Design review of the part built by this model. Coordinates are the model's own, in mm. Face numbers are marked on the shaded views. Coordinates: 2 decimals unless noted, no trailing zeros. Loops run counter-clockwise (first coordinate to the right, second up) from the corner with the lowest first, then second, coordinate; pieces in that order, holes last.
Q1. Wall thickness on probe 1 along X at (y, z) = (14.2, 0); probe 2 along Y at (x, z) = (13, 10.5); probe 3 along X at (y, z) = (11.05, -27.5): over which ranges is each line inside the solid? List them lowest first.
Q2. Add section D-D on x = -27.5. Give the boundary of the cut face in (y, z), and give its area (3 significant figures).
Q3. Add section B-B on x = 0. Give the boundary of the cut face in (y, z), and give its area (4 significant figures).
Q4. Add section A-A on z = -27.5. Give the boundary of the cut face in (x, y), and give its area (3 significant figures).
Q5. For P1, Ø4, axis at x = 0, z = 27.5, coming from the -Y side; P2, Ø1.5, axis at y = 2.5, z = -17.5, coming from the +X side; P3, Ø12, axis at x = 8, z = -24.5, coming from the +Y side, all flat-tipped, find the tip position at first contact; note any pin that passes through.
Q6. Draft analysis for pull direction Z (two halves, no side actions). For the marked faces 1 and 2, state which applies: released by +Z, released by -Z, zero draft, split by the parting line, or undercut.
Q7. Add section C-C on z = 0. Give the boundary of the cut face in (x, y), and give its area (4 significant figures).
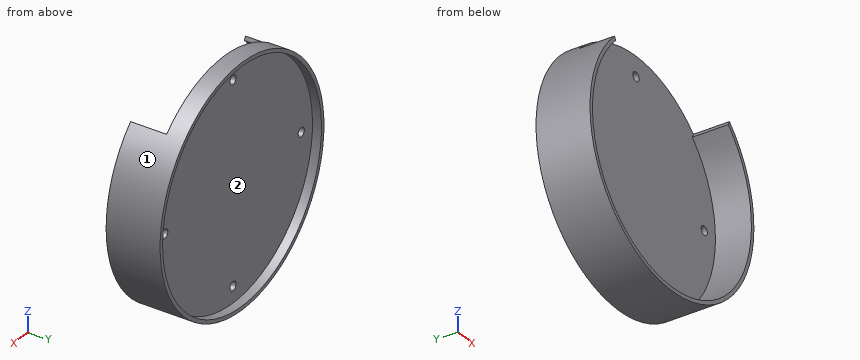
```python
from build123d import *

# Parameters (mm, degrees)
SKETCH1_R               = 33
SKETCH1_R_2             = 1.25
BOSS_EXTRUDE1_DEPTH     = 12.5
SKETCH2_R               = 32
CUT_EXTRUDE2_DEPTH      = 10
SKETCH8_R               = 33
SKETCH8_R_2             = 32
BOSS_EXTRUDE2_DEPTH     = 15
CUT_REVOLVE_THIN2_DEPTH = 10


# Read off the part's stored shape, not the designer's step: Cut-Revolve-Thin2
with BuildPart() as part:
    # Sketch1 → Boss-Extrude1 (new body)
    with BuildSketch(Plane(origin=(0, 0, 0), x_dir=(1, 0, 0), z_dir=(0, 1, 0))):
        with Locations(Location((0, 0, 0), (0, 0, 270))):
            Circle(SKETCH1_R)
        with Locations(Location((0, 27.5, 0), (0, 0, 270))):
            Circle(SKETCH1_R_2, mode=Mode.SUBTRACT)
        with Locations(Location((27.5, 0, 0), (0, 0, 270))):
            Circle(SKETCH1_R_2, mode=Mode.SUBTRACT)
        with Locations(Location((0, -27.5, 0), (0, 0, 270))):
            Circle(SKETCH1_R_2, mode=Mode.SUBTRACT)
        with Locations(Location((-27.5, 0, 0), (0, 0, 270))):
            Circle(SKETCH1_R_2, mode=Mode.SUBTRACT)
    extrude(amount=BOSS_EXTRUDE1_DEPTH)

    # Sketch2 → Cut-Extrude2 (cut)
    with BuildSketch(Plane(origin=(0, 0, 0), x_dir=(1, 0, 0), z_dir=(0, 1, 0))):
        with Locations(Location((0, 0, 0), (0, 0, 270))):
            Circle(SKETCH2_R)
    extrude(amount=CUT_EXTRUDE2_DEPTH, mode=Mode.SUBTRACT)

    # Sketch8 → Boss-Extrude2 (add)
    with BuildSketch(Plane(origin=(0, 0, 0), x_dir=(1, 0, 0), z_dir=(0, 1, 0))):
        with Locations(Location((0, 0, 0), (0, 0, 270))):
            Circle(SKETCH8_R)
        with Locations(Location((0, 0, 0), (0, 0, 270))):
            Circle(SKETCH8_R_2, mode=Mode.SUBTRACT)
    extrude(amount=BOSS_EXTRUDE2_DEPTH)

    # Cut-Revolve-Thin2 outline → Cut-Revolve-Thin2 (cut)
    with BuildSketch(Plane(origin=(0, 0, 0), x_dir=(1, 0, 0), z_dir=(0, 1, 0))):
        with BuildLine():
            ThreePointArc((-22.709083631, -22.545454545), (-22.928374212, -23.0355805), (-23.137087961, -23.53030303))
            ThreePointArc((-23.137087961, -23.53030303), (0, -33), (23.137087961, -23.53030303))
            ThreePointArc((23.137087961, -23.53030303), (22.928374212, -23.0355805), (22.709083631, -22.545454545))
            ThreePointArc((22.709083631, -22.545454545), (0, -32), (-22.709083631, -22.545454545))
        make_face()
    extrude(amount=CUT_REVOLVE_THIN2_DEPTH, mode=Mode.SUBTRACT)


solid = part.part
```
Entries:
1. probe 1: x = -33 to -32, 32 to 33
1. probe 2: y = 10 to 12.5
1. probe 3: x = -18.24 to -1.25, 1.25 to 18.24
2. outline: (0, -18.24) - (15, -18.24) - (15, -16.36) - (12.5, -16.36) - (12.5, -1.25) - (10, -1.25) - (10, -16.36) - (0, -16.36) - close; (0, 16.36) - (10, 16.36) - (10, 1.25) - (12.5, 1.25) - (12.5, 16.36) - (15, 16.36) - (15, 18.24) - (0, 18.24) - close
2. area: 132 mm2
3. outline: (0, -33) - (15, -33) - (15, -32) - (12.5, -32) - (12.5, -28.75) - (10, -28.75) - (10, -32) - (0, -32) - close; (10, -26.25) - (12.5, -26.25) - (12.5, 26.25) - (10, 26.25) - close; (10, 28.75) - (12.5, 28.75) - (12.5, 32) - (15, 32) - (15, 33) - (10, 33) - close
3. area: 167.5 mm2
4. outline: (-18.24, 0) - (-16.36, 0) - (-16.36, 10) - (-1.25, 10) - (-1.25, 12.5) - (-16.36, 12.5) - (-16.36, 15) - (-18.24, 15) - close; (1.25, 10) - (16.36, 10) - (16.36, 0) - (18.24, 0) - (18.24, 15) - (16.36, 15) - (16.36, 12.5) - (1.25, 12.5) - close
4. area: 132 mm2
5. P1: stops at y = 10
5. P2: stops at x = 28.43
5. P3: stops at y = 12.5
6. face 1: split by the parting line
6. face 2: undercut
7. outline: (-33, 0) - (-32, 0) - (-32, 10) - (-28.75, 10) - (-28.75, 12.5) - (-32, 12.5) - (-32, 15) - (-33, 15) - close; (-26.25, 10) - (26.25, 10) - (26.25, 12.5) - (-26.25, 12.5) - close; (28.75, 10) - (32, 10) - (32, 0) - (33, 0) - (33, 15) - (32, 15) - (32, 12.5) - (28.75, 12.5) - close
7. area: 177.5 mm2
